Input: part model. Units: mm. Frame: model coordinates. Face numbers are marked on the shaded views. A direction names the side the tool comes from. Give positions to 0.01 mm unless a question says otherwise; leave off trailing zeros. Loops run counter-clockwise (first coordinate to the right, second up) from the corner with the lowest first, then second, coordinate; pieces in that order, holes last. Notation, with made-up numbers: M 54.25,-4.5 L 92.25,-4.5 A27 cw 92.25,33.5 Z; hole C -31,-4.75 d6. An arc over 180 degrees is marked long. Answer as a JSON object with one key per item and string values. Group by question number.
```python
from build123d import *

# Parameters (mm, degrees)
F1_DEPTH = 22.606
F3_DEPTH = 56.642
F5_DEPTH = 123.952
F6_W     = 17.9281285021
F6_H     = 3.7313278299
F7_DEPTH = 131.318
F8_SIZE  = 1.27


with BuildPart() as f1:
    # F0 (on Top) → F1 (new body)
    with BuildSketch(Plane.XY):
        Polygon((67.9795068204, -48.892733641), (67.9795068204, -23.492733641), (-59.0204931796, -23.492733641), (-59.0204931796, -41.780733641), (-57.7496923506, -41.780733641), (-57.7496923506, -48.892733641), (-57.7496923506, -56.004733641), (-59.0204931796, -56.004733641), (-59.0204931796, -74.292733641), (67.9795068204, -74.292733641), align=None)
    extrude(amount=F1_DEPTH)

    # F2 (on face) → F3 (cut)
    with BuildSketch(Plane.XZ.offset(74.292733641)):
        Polygon((-59.0204931796, 22.606), (-59.0204931796, 7.1184414792), (-58.0175313886, 12.4418523751), (-43.2899855077, 22.606), align=None)
        with BuildLine():
            Line((55.4608365675, 1.4634394883), (-49.7719274679, 1.4634394883))
            Line((-49.7719274679, 1.4634394883), (-57.9830260793, 5.7754135323))
            Line((-57.9830260793, 5.7754135323), (-59.0204931796, 6.0288892267))
            Line((-59.0204931796, 6.0288892267), (-59.0204931796, 0))
            Line((-59.0204931796, 0), (67.9795068204, 0))
            Line((67.9795068204, 0), (67.9795068204, 22.606))
            Line((67.9795068204, 22.606), (58.8168874383, 22.606))
            Line((58.8168874383, 22.606), (67.5153278326, 10.7161320989))
            Line((67.5153278326, 10.7161320989), (67.1798294962, 8.7120201094))
            Line((67.1798294962, 8.7120201094), (63.0014389753, 1.7273251433))
            add(Edge.make_bspline(
                [(55.4608365675, 1.4634394883), (55.7992606547, 1.1248105944), (56.5402688521, 0.3862817839), (58.6439188352, -0.0157318094), (60.613555974, 0.3869426535), (61.8581460025, 1.1113634898), (62.6646578312, 1.4950803015), (63.0014389753, 1.7273251433)],
                knots=[0, 0, 0, 0, 0.1896033215, 0.4147497426, 0.6360801274, 0.8233787666, 1, 1, 1, 1], degree=3))
        make_face()
    extrude(amount=-F3_DEPTH, mode=Mode.SUBTRACT)

    # F4 (on face) → F5 (cut)
    with BuildSketch(Plane(origin=(-57.7496923506, 0, 0), x_dir=(0, -1, 0), z_dir=(-1, 0, 0))):
        Polygon((39.9286693899, 5.5741476826), (24.2253392935, 5.5741476826), (24.2253392935, 0.5848236615), (24.2253392935, -3.517596783), (39.9286693899, -3.517596783), (39.9286693899, 0.5848236615), align=None)
        Polygon((73.5601279885, 5.5741476826), (57.856797892, 5.5741476826), (57.856797892, 0.5848236615), (57.856797892, -3.517596783), (73.5601279885, -3.517596783), (73.5601279885, 0.5848236615), align=None)
    extrude(amount=-F5_DEPTH, mode=Mode.SUBTRACT)

    # F6 (on face) → F7 (cut)
    with BuildSketch(Plane(origin=(-57.7496923506, 0, 0), x_dir=(0, -1, 0), z_dir=(-1, 0, 0))):
        with Locations((48.892733641, -0.1383387716)):
            Rectangle(F6_W, F6_H)
    extrude(amount=-F7_DEPTH, mode=Mode.SUBTRACT)

    # F8
    f8_edges = [f1.edges().sort_by_distance(p)[0] for p in [
        (-50.653758, -23.492734, 17.523926),
        (-50.653758, -74.292734, 17.523926),
        (7.763451, -23.492734, 22.606),
        (7.763451, -74.292734, 22.606),
        (63.166108, -74.292734, 16.661066),
        (63.166108, -23.492734, 16.661066),
    ]]
    chamfer(f8_edges, length=F8_SIZE)


solid = f1.part
```
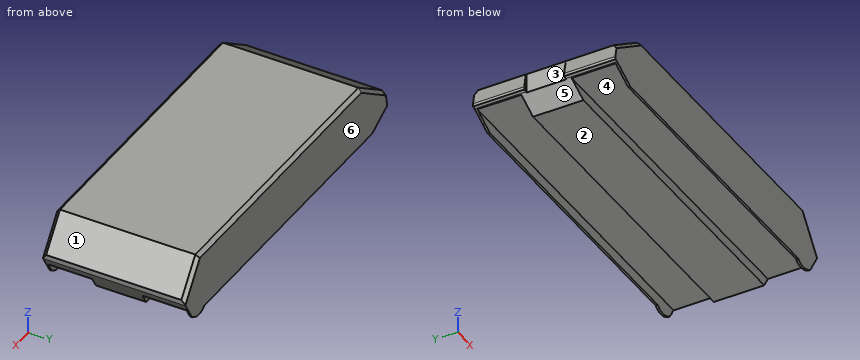
1. First-contact query: P1, Ø8, axis at x = -23.5, y = -31, coming from the -Z side; P2, Ø3.5, axis at y = -49.5, z = 10.5, coming from the -X side; P3, Ø6, axis at y = -58, z = 13, coming from the -X side. Flat tips, straight axial feed; report the tip coordinate or a pass-through.
2. Section C-C (x = 29.5). Output: boundary loops of the cut face in (y, z).
3. Section A-A (y = -59). Output: boundary loops of the cut face in (x, z).
4. Reachability of the marked faces 1, 2 and 3 from +Z, -Z, +X, -X, +Y, -Y: full face, straight path, thin tool, end or side. Return the list, or none.
5. Mould query, pull axis Y, two halves, no side actions, for the marked faces 4, 5 and 6. Classes: pulls with the +Y half, pulls with the -Y half, needs draft (parallel to the pull), parting line crosses it, or undercut.
6. Section D-D (z = 19). Output: boundary loops of the cut face in (x, y), then the cut area to 3 significant figures.
7. Section B-B (z = 4.25). Output: boundary loops of the cut face in (x, y).
8. Material intervals for L1, parallel to Y at x = 30, z = 2; L2, parallel to Z at x = -41, y = -36.5; L3, parallel to Z at x = 58, y = -40, sorted ascending.
Geometry results:
{
 "1": {"P1": "z = 5.57", "P2": "x = -57.75", "P3": "x = -58.48"},
 "2": {"outline": "M -74.29,1.46 L -73.56,1.46 L -73.56,5.57 L -57.86,5.57 L -57.86,1.73 L -39.93,1.73 L -39.93,5.57 L -24.23,5.57 L -24.23,1.46 L -23.49,1.46 L -23.49,21.34 L -24.76,22.61 L -73.02,22.61 L -74.29,21.34 Z"},
 "3": {"outline": "M -59.02,6.03 L -57.98,5.78 L -57.6,5.57 L 65.3,5.57 L 67.18,8.71 L 67.52,10.72 L 58.82,22.61 L -43.29,22.61 L -58.02,12.44 L -59.02,7.12 Z"},
 "4": {"face 1": "+Z, +X, +Y, -Y", "face 2": "-Z, +X, -X", "face 3": "+Z, -Z, -X"},
 "5": {"face 4": "undercut", "face 5": "needs draft", "face 6": "pulls with the +Y half"},
 "6": {"outline": "M -48.51,-73.02 L -46.28,-74.29 L 59.88,-74.29 L 61.45,-73.02 L 61.45,-24.76 L 59.88,-23.49 L -46.28,-23.49 L -48.51,-24.76 Z", "area": "5,580 mm2"},
 "7": {"outline": "M -55.08,-74.29 L 64.51,-74.29 L 64.51,-73.56 L -55.08,-73.56 Z; M -55.08,-57.86 L 64.51,-57.86 L 64.51,-39.93 L -55.08,-39.93 Z; M -55.08,-24.23 L 64.51,-24.23 L 64.51,-23.49 L -55.08,-23.49 Z"},
 "8": {"L1": "-74.29 to -73.56, -57.86 to -39.93, -24.23 to -23.49", "L2": "5.57 to 22.61", "L3": "1.73 to 22.61"}
}
